Could you check a few things on this model? Use its own coordinates, in mm. A direction names the side the tool comes from. Round coordinates to 2 decimals unless told otherwise and drop trailing zeros. Loops run counter-clockwise (first coordinate to the right, second up) from the corner with the lowest first, then second, coordinate; pieces in that order, holes last. Notation, with made-up numbers: M 17.25,21 L 45.25,21 A27 ccw 45.25,37 Z; hole C 87,80 d8. An arc over 180 degrees is marked long. Answer in a Markdown table with one row per item.
```python
from build123d import *

# Parameters (mm, degrees)
BOSS_EXTRUDE1_DEPTH = 10
SKETCH4_R           = 2
CUT_EXTRUDE1_DEPTH  = 5


with BuildPart() as part:
    # Sketch3 → Boss-Extrude1 (new body)
    with BuildSketch(Plane(origin=(0, 0, 0), x_dir=(0, 0, -1), z_dir=(1, 0, 0))):
        Polygon((18.594382672, 46.957725761), (18.594382672, -5.042274239), (-141.405617328, -5.042274239), (-141.405617328, 36.957725761), (-46.405617328, 46.957725761), align=None)
    extrude(amount=BOSS_EXTRUDE1_DEPTH)

    # Sketch4 → Cut-Extrude1 (cut)
    with BuildSketch(Plane(origin=(10, 0, 0), x_dir=(0, 0, -1), z_dir=(1, 0, 0))):
        with Locations((-136.405617328, 31.957725761)):
            Circle(SKETCH4_R)
        with Locations((-136.405617328, 3.957725761)):
            Circle(SKETCH4_R)
        with Locations((13.594382672, 3.957725761)):
            Circle(SKETCH4_R)
        with Locations((13.594382672, 31.957725761)):
            Circle(SKETCH4_R)
    extrude(amount=-CUT_EXTRUDE1_DEPTH, mode=Mode.SUBTRACT)


solid = part.part
```
1) Will these pins go through, and if not, where does the flat tip stop? P1, Ø1, axis at x = 4.5, z = 116.5, coming from the +Y side; P2, Ø3, axis at y = 31.96, z = 136.41, coming from the +X side.
Computed:
| item | result |
|---|---|
| P1 | stops at y = 39.63 |
| P2 | stops at x = 5 |
2) I want a section at B-B, the plane z = 91. Please give me the cut outline in (x, y).
Computed:
| item | result |
|---|---|
| outline | M 0,-5.04 L 10,-5.04 L 10,42.26 L 0,42.26 Z |
3) If we mould it in two halves opening along Z, with no side actions, what happens to faces 3 (the face through (5, -5.042, 60)), 4 (the face through (7.54, 33.94, 136.67)), 5 (the face through (5, 16, 141.406))? For each: released by +Z, released by -Z, zero draft, split by the parting line, or undercut.
Computed:
| item | result |
|---|---|
| face 3 | zero draft |
| face 4 | undercut |
| face 5 | released by +Z |
4) I want a section at A-A, the plane x = 6.75. Please give me the cut outline in (y, z), plus the area to 3 significant figures.
Computed:
| item | result |
|---|---|
| outline | M -5.04,-18.59 L 46.96,-18.59 L 46.96,46.41 L 36.96,141.41 L -5.04,141.41 Z; hole C 3.96,-13.59 d4; hole C 3.96,136.41 d4; hole C 31.96,-13.59 d4; hole C 31.96,136.41 d4 |
| area | 7,790 mm² |
5) Which directions (+Z, -Z, +X, -X, +Y, -Y) give clear straight access to the entire face, cutting with the end or side of a thin tool? Please do faces 1 (the face through (7.535, 33.644, -14.67)), 2 (the face through (5, 21, -18.594)).
Computed:
| item | result |
|---|---|
| face 1 | +X |
| face 2 | -Z, +X, -X, +Y, -Y |
6) I need wall thicknesses on line 1 (Y direction, x = 6.25, z = 97); line 2 (Y direction, x = 5, z = 63). Which ranges of each line are inside material? Lowest first, please.
Computed:
| item | result |
|---|---|
| line 1 | y = -5.04 to 41.63 |
| line 2 | y = -5.04 to 45.21 |
7) I want a section at C-C, the plane z = 119. Please give me the cut outline in (x, y).
Computed:
| item | result |
|---|---|
| outline | M 0,-5.04 L 10,-5.04 L 10,39.32 L 0,39.32 Z |
